Design review of the part built by this model. Coordinates are the model's own, in mm. Coordinates: 2 decimals unless noted, no trailing zeros. Write each loop counter-clockwise with the first axis right and the second up, starting at its lowest first coordinate (ties: lowest second). Pieces come first, ordered by that corner, then holes.
Q1. For probe 1 along Y at (x, z) = (-30, 8.75); probe 2 along Z at (x, y) = (-50, -197); probe 3 along Y at (x, z) = (66.5, 6.25), list the stretches that pass through material, from the lowest coordinate up.
Q2. Insertion check: pin 1 (4.5 mm diameter, centred on x = -111.5, z = 11.5, fed in from +Y); pin 2 (6 mm diameter, centred on y = -85, z = 15.5, fed in from -X); pin 3 (5.5 mm diameter, centred on x = -114.5, z = 11, fed in from -Y). Each pin has a flat end and moves straight along its axis. Give the tip position at first contact, or say it passes through.
Q3. Take a section at A-A (y = -83.5). Give the boundary of the cut face in (x, z), and give its area (3 significant figures).
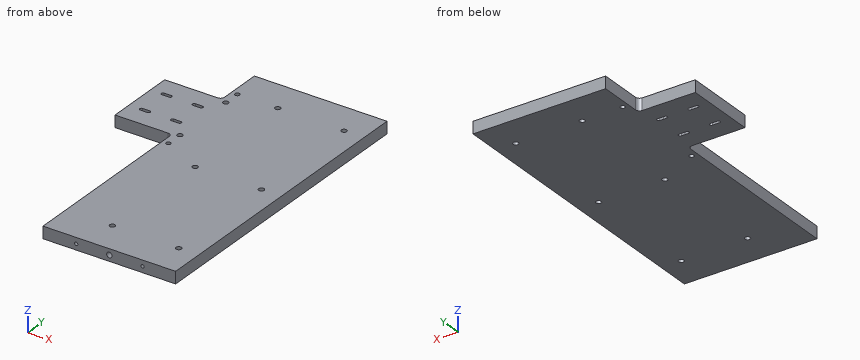
```python
from build123d import *

# Parameters (mm, degrees)
SKETCH1_W                   = 200
SKETCH1_H                   = 460
BOSS_EXTRUDE1_DEPTH         = 18
OTWORY_USTALAJ_CE_8_0MM1_D  = 8
OTW_R_7_0_7_1_D             = 7
OTW_R_5_0_5_1_D             = 5
OTW_R_5_0_5_1_DEPTH         = 45
OTW_R_5_0_5_1_TIP           = 1.502151548
DODANIE_WYCI_GNI_CIE1_DEPTH = 18
OTW_R_5_0_5_2_D             = 5
WYTNIJ_WYCI_GNI_CIE1_DEPTH  = 297.344394244
OTW_R_8_0_8_1_D             = 8
OTW_R_8_0_8_1_DEPTH         = 15
OTW_R_8_0_8_1_TIP           = 2.403442476
OTW_R_8_0_8_2_D             = 8
OTW_R_8_0_8_2_DEPTH         = 22
OTW_R_8_0_8_2_TIP           = 2.403442476


with BuildPart() as part:
    # Sketch1 → Boss-Extrude1 (new body)
    with BuildSketch(Plane.XY):
        Rectangle(SKETCH1_W, SKETCH1_H)
    extrude(amount=BOSS_EXTRUDE1_DEPTH)

    # Otwory ustalające Ø8.0mm1 (through all)
    with Locations(Plane(origin=(0, 0, 0), x_dir=(-1, 0, 0), z_dir=(0, 0, -1))):
        with Locations((-70, 180), (-70, 0), (-70, -180), (30, -180), (30, 0), (30, 180)):
            Hole(OTWORY_USTALAJ_CE_8_0MM1_D / 2)

    # Otwór Ø7.0 (7)1 (through all)
    with Locations(Plane.XY.offset(18)):
        with Locations((-91, 180), (-91, 30)):
            Hole(OTW_R_7_0_7_1_D / 2)

    # Otwór Ø5.0 (5)1
    with Locations(Plane(origin=(0, -230, 0), x_dir=(-1, 0, 0), z_dir=(0, -1, 0))):
        with Locations((50, -9), (-50, -9)):
            Hole(OTW_R_5_0_5_1_D / 2, depth=OTW_R_5_0_5_1_DEPTH)
            with Locations((0, 0, -(OTW_R_5_0_5_1_DEPTH + OTW_R_5_0_5_1_TIP / 2))):  # 118° drill point
                Cone(0, OTW_R_5_0_5_1_D / 2, OTW_R_5_0_5_1_TIP, mode=Mode.SUBTRACT)

    # Szkic8 → Dodanie-wyciągnięcie1 (add)
    with BuildSketch(Plane.XY.offset(18)):
        with BuildLine():
            Line((-100, 165), (-100, 45))
            ThreePointArc((-100, 45), (-101.757359313, 49.242640687), (-106, 51))
            Line((-106, 51), (-186, 51))
            Line((-186, 51), (-186, 159))
            Line((-186, 159), (-106, 159))
            ThreePointArc((-106, 159), (-101.757359313, 160.757359313), (-100, 165))
        make_face()
    extrude(amount=-DODANIE_WYCI_GNI_CIE1_DEPTH)

    # Otwór Ø5.0 (5)2 (through all)
    with Locations(Plane.XY.offset(18)):
        with Locations((-161.928446298, 128.5), (-114.928446334, 128.498158688), (-114.928446334, 81.498158688), (-161.928446298, 81.5)):
            Hole(OTW_R_5_0_5_2_D / 2)

    # Szkic11 → Wytnij-wyciągnięcie1 (cut, through all)
    with BuildSketch(Plane(origin=(0, 0, 0), x_dir=(-1, 0, 0), z_dir=(0, 0, -1))):
        with BuildLine():
            Line((109.5, 131), (120.5, 131))
            ThreePointArc((120.5, 131), (123, 128.5), (120.5, 126))
            Line((120.5, 126), (109.5, 126))
            ThreePointArc((109.5, 126), (107, 128.5), (109.5, 131))
        make_face()
        with BuildLine():
            Line((156.5, 131), (167.5, 131))
            ThreePointArc((167.5, 131), (170, 128.5), (167.5, 126))
            Line((167.5, 126), (156.5, 126))
            ThreePointArc((156.5, 126), (154, 128.5), (156.5, 131))
        make_face()
        with BuildLine():
            Line((109.5, 84), (120.5, 84))
            ThreePointArc((120.5, 84), (123, 81.5), (120.5, 79))
            Line((120.5, 79), (109.5, 79))
            ThreePointArc((109.5, 79), (107, 81.5), (109.5, 84))
        make_face()
        with BuildLine():
            Line((156.5, 84), (167.5, 84))
            ThreePointArc((167.5, 84), (170, 81.5), (167.5, 79))
            Line((167.5, 79), (156.5, 79))
            ThreePointArc((156.5, 79), (154, 81.5), (156.5, 84))
        make_face()
    extrude(amount=-WYTNIJ_WYCI_GNI_CIE1_DEPTH, mode=Mode.SUBTRACT)

    # Otwór Ø8.0 (8)1
    with Locations(Plane.XY.offset(18)):
        with Locations((-91, 155), (-91, 55)):
            Hole(OTW_R_8_0_8_1_D / 2, depth=OTW_R_8_0_8_1_DEPTH)
            with Locations((0, 0, -(OTW_R_8_0_8_1_DEPTH + OTW_R_8_0_8_1_TIP / 2))):  # 118° drill point
                Cone(0, OTW_R_8_0_8_1_D / 2, OTW_R_8_0_8_1_TIP, mode=Mode.SUBTRACT)

    # Otwór Ø8.0 (8)2
    with Locations(Plane(origin=(0, -230, 0), x_dir=(-1, 0, 0), z_dir=(0, -1, 0))):
        with Locations((0, -9)):
            Hole(OTW_R_8_0_8_2_D / 2, depth=OTW_R_8_0_8_2_DEPTH)
            with Locations((0, 0, -(OTW_R_8_0_8_2_DEPTH + OTW_R_8_0_8_2_TIP / 2))):  # 118° drill point
                Cone(0, OTW_R_8_0_8_2_D / 2, OTW_R_8_0_8_2_TIP, mode=Mode.SUBTRACT)


solid = part.part
```
Response:
1. probe 1: y = -230 to -184, -176 to -4, 4 to 176, 184 to 230
1. probe 2: z = 0 to 6.5, 11.5 to 18
1. probe 3: y = -230 to -181.94, -178.06 to -1.94, 1.94 to 178.06, 181.94 to 230
2. pin 1: stops at y = 159
2. pin 2: stops at x = -100
2. pin 3: stops at y = 51
3. outline: (-100, 0) - (100, 0) - (100, 18) - (-100, 18) - close
3. area: 3,600 mm2
